```python
from build123d import *

# Parameters (mm, degrees)
SKETCH1_W                = 75
SKETCH1_H                = 110
BOSS_EXTRUDE1_DEPTH      = 3
SKETCH2_W                = 3
SKETCH2_H                = 10
CUT_EXTRUDE1_DEPTH       = 3
M3_CLEARANCE_HOLE1_D     = 3.4
M3_CLEARANCE_HOLE1_DEPTH = 3
M3_CLEARANCE_HOLE1_TIP   = 1.021463052


with BuildPart() as part:
    # Sketch1 → Boss-Extrude1 (new body)
    with BuildSketch(Plane(origin=(0, 0, 0), x_dir=(1, 0, 0), z_dir=(0, 1, 0))):
        with Locations((37.5, 55)):
            Rectangle(SKETCH1_W, SKETCH1_H)
    extrude(amount=BOSS_EXTRUDE1_DEPTH)

    # Sketch2 → Cut-Extrude1 (cut)
    with BuildSketch(Plane(origin=(0, 3, 0), x_dir=(1, 0, 0), z_dir=(0, 1, 0))):
        with Locations((6.5, 91)):
            Rectangle(SKETCH2_W, SKETCH2_H)
        with Locations((68.5, 91)):
            Rectangle(SKETCH2_W, SKETCH2_H)
        with Locations((68.5, 20)):
            Rectangle(SKETCH2_W, SKETCH2_H)
        with Locations((6.5, 20)):
            Rectangle(SKETCH2_W, SKETCH2_H)
        with Locations((19, 65)):
            Rectangle(SKETCH2_W, SKETCH2_H)
    extrude(amount=-CUT_EXTRUDE1_DEPTH, mode=Mode.SUBTRACT)

    # M3 Clearance Hole1
    with Locations(Plane(origin=(0, 3, 0), x_dir=(1, 0, 0), z_dir=(0, 1, 0))):
        with Locations((6.5, 10), (68.5, 10), (19, 55)):
            Hole(M3_CLEARANCE_HOLE1_D / 2, depth=M3_CLEARANCE_HOLE1_DEPTH)
            with Locations((0, 0, -(M3_CLEARANCE_HOLE1_DEPTH + M3_CLEARANCE_HOLE1_TIP / 2))):  # 118° drill point
                Cone(0, M3_CLEARANCE_HOLE1_D / 2, M3_CLEARANCE_HOLE1_TIP, mode=Mode.SUBTRACT)


solid = part.part
```
Design review of the part built by this model. Coordinates are the model's own, in mm. A direction names the side the tool comes from. Round coordinates to 2 decimals unless told otherwise and drop trailing zeros. Write each loop counter-clockwise with the first axis right and the second up, starting at its lowest first coordinate (ties: lowest second). Pieces come first, ordered by that corner, then holes. Notation, with made-up numbers: (38, -5) -> (50, -5) arc R11 cw to (50, 13) -> close; hole circle Ø4 at (15.5, 79.5). An arc over 180 degrees is marked (long way). Answer in a Markdown table with one row per item.
Q1. Take a section at C-C, the plane y = 1.15. Count the separate pieces of the cut face and the enclosed holes in it, then the cut area to 3 significant figures.
The answers:
| item | result |
|---|---|
| separate pieces | 1 |
| enclosed holes | 8 |
| area | 8,070 mm² |
Q2. Draft analysis for pull direction X (two halves, no side actions). For faces 3 (the face through (5, 2, -20)), 4 (the face through (37, 0, -56)), 5 (the face through (0, 1, -54)), state which applies: +X half, -X half, draft (parallel to the pull), parting line (faces both ways), or undercut.
The answers:
| item | result |
|---|---|
| face 3 | undercut |
| face 4 | draft |
| face 5 | -X half |
Q3. Take a section at B-B, the plane x = 6.5. State the section outline as (y, z) points, then the cut area to 3 significant figures.
The answers:
| item | result |
|---|---|
| outline | (0, -110) -> (3, -110) -> (3, -96) -> (0, -96) -> close; (0, -86) -> (3, -86) -> (3, -25) -> (0, -25) -> close; (0, -15) -> (3, -15) -> (3, -11.7) -> (0, -11.7) -> close; (0, -8.3) -> (3, -8.3) -> (3, 0) -> (0, 0) -> close |
| area | 260 mm² |
Q4. Clearance check with a flat-ended pin moving along its axis: pin 1 Ø2.5 at (x, z) = (19, -55) entering from -Y (3 decimals). State where the tip first meets the part, or that it passes through.
The answers:
| item | result |
|---|---|
| pin 1 | through |
Q5. Take a section at D-D, the plane z = -17.5. State the section outline as (x, y) points.
The answers:
| item | result |
|---|---|
| outline | (0, 0) -> (5, 0) -> (5, 3) -> (0, 3) -> close; (8, 0) -> (67, 0) -> (67, 3) -> (8, 3) -> close; (70, 0) -> (75, 0) -> (75, 3) -> (70, 3) -> close |
Q6. For faces 1 (the face through (6, 2, -15)), 2 (the face through (37, 1, 0)), list the 3-axis set-ups (+Z, -Z, +X, -X, +Y, -Y) from which the entire face can be reached by the end or side of a thin tool; tool diameter is ignored.
The answers:
| item | result |
|---|---|
| face 1 | +Y, -Y |
| face 2 | +Z, +X, -X, +Y, -Y |
Q7. To check wall thickness, follow L1, parallel to Z at x = 6.5, y = 1.35; L2, parallel to Z at x = 19, y = 1.1; L3, parallel to X at y = 1, z = -10. State the ranges of each line that lie inside material, in increasing order. Write a range as [from, to].
The answers:
| item | result |
|---|---|
| L1 | [-110, -96], [-86, -25], [-15, -11.7], [-8.3, 0] |
| L2 | [-110, -70], [-60, -56.7], [-53.3, 0] |
| L3 | [0, 4.8], [8.2, 66.8], [70.2, 75] |
Q8. Take a section at A-A, the plane z = -55. State the section outline as (x, y) points.
The answers:
| item | result |
|---|---|
| outline | (0, 0) -> (17.3, 0) -> (17.3, 3) -> (0, 3) -> close; (20.7, 0) -> (75, 0) -> (75, 3) -> (20.7, 3) -> close |
